The model under review builds one solid part; all positions refer to its coordinate system, in mm. A direction names the side the tool comes from. Give positions to 0.01 mm unless a question says otherwise; leave off trailing zeros. Loops run counter-clockwise (first coordinate to the right, second up) from the corner with the lowest first, then second, coordinate; pieces in that order, holes last. Notation, with made-up numbers: (8.25, -11) - (44.25, -11) arc R17 cw to (44.25, 9) - close; hole circle Ø4 at (-30.75, -3). An arc over 180 degrees is marked (long way). Return JSON: item names as keys, results as strings. Group by question number.
```python
from build123d import *

# Parameters (mm, degrees)
SKETCH1_W           = 172
SKETCH1_H           = 222
SKETCH1_R           = 1.55
SKETCH1_W_2         = 50
SKETCH1_H_2         = 10
BOSS_EXTRUDE2_DEPTH = 4
FILLET1_R           = 4


with BuildPart() as part:
    # Sketch1 → Boss-Extrude2 (new body)
    with BuildSketch(Plane(origin=(0, 0, 0), x_dir=(0, 1, 0), z_dir=(0, 0, 1))):
        with Locations((86, 111)):
            Rectangle(SKETCH1_W, SKETCH1_H)
        with Locations(Location((5, 4, 0), (0, 0, 270))):
            Circle(SKETCH1_R, mode=Mode.SUBTRACT)
        with Locations(Location((5, 218, 0), (0, 0, 270))):
            Circle(SKETCH1_R, mode=Mode.SUBTRACT)
        with Locations(Location((167, 218, 0), (0, 0, 270))):
            Circle(SKETCH1_R, mode=Mode.SUBTRACT)
        with Locations(Location((167, 4, 0), (0, 0, 270))):
            Circle(SKETCH1_R, mode=Mode.SUBTRACT)
        with Locations(Location((86, 218, 0), (0, 0, 270))):
            Circle(SKETCH1_R, mode=Mode.SUBTRACT)
        with Locations(Location((86, 4, 0), (0, 0, 270))):
            Circle(SKETCH1_R, mode=Mode.SUBTRACT)
        with Locations(Location((4, 61, 0), (0, 0, 270))):
            Circle(SKETCH1_R, mode=Mode.SUBTRACT)
        with Locations(Location((168, 61, 0), (0, 0, 270))):
            Circle(SKETCH1_R, mode=Mode.SUBTRACT)
        with Locations(Location((168, 161, 0), (0, 0, 270))):
            Circle(SKETCH1_R, mode=Mode.SUBTRACT)
        with Locations(Location((4, 161, 0), (0, 0, 270))):
            Circle(SKETCH1_R, mode=Mode.SUBTRACT)
        with Locations((55, 207)):
            Rectangle(SKETCH1_W_2, SKETCH1_H_2, mode=Mode.SUBTRACT)
        with Locations((55, 15)):
            Rectangle(SKETCH1_W_2, SKETCH1_H_2, mode=Mode.SUBTRACT)
        with BuildLine():
            Line((40, 131), (40, 91))
            ThreePointArc((40, 91), (35, 86), (30, 91))
            Line((30, 91), (30, 131))
            ThreePointArc((30, 131), (35, 136), (40, 131))
        make_face(mode=Mode.SUBTRACT)
        with BuildLine():
            Line((60, 131), (60, 91))
            ThreePointArc((60, 91), (55, 86), (50, 91))
            Line((50, 91), (50, 131))
            ThreePointArc((50, 131), (55, 136), (60, 131))
        make_face(mode=Mode.SUBTRACT)
        with BuildLine():
            Line((80, 131), (80, 91))
            ThreePointArc((80, 91), (75, 86), (70, 91))
            Line((70, 91), (70, 131))
            ThreePointArc((70, 131), (75, 136), (80, 131))
        make_face(mode=Mode.SUBTRACT)
        with BuildLine():
            Line((100, 131), (100, 91))
            ThreePointArc((100, 91), (95, 86), (90, 91))
            Line((90, 91), (90, 131))
            ThreePointArc((90, 131), (95, 136), (100, 131))
        make_face(mode=Mode.SUBTRACT)
        with BuildLine():
            Line((120, 131), (120, 91))
            ThreePointArc((120, 91), (115, 86), (110, 91))
            Line((110, 91), (110, 131))
            ThreePointArc((110, 131), (115, 136), (120, 131))
        make_face(mode=Mode.SUBTRACT)
        with BuildLine():
            Line((140, 131), (140, 91))
            ThreePointArc((140, 91), (135, 86), (130, 91))
            Line((130, 91), (130, 131))
            ThreePointArc((130, 131), (135, 136), (140, 131))
        make_face(mode=Mode.SUBTRACT)
    extrude(amount=BOSS_EXTRUDE2_DEPTH)

    # Fillet1
    # the kernel refuses this fillet: 4 mm, written as the material it takes off along each edge
    with BuildSketch(Plane(origin=(10, 172, 0), x_dir=(0, 0, 1), z_dir=(-1, 0, 0)), Plane(origin=(-232, 0, 0), x_dir=(0, 0, 1), z_dir=(1, 0, 0))) as fillet1_piece_1:
        with BuildLine():
            CenterArc((FILLET1_R, -FILLET1_R), FILLET1_R, 90, 90)
            Line((0, -FILLET1_R), (0, 0))
            Line((0, 0), (FILLET1_R, 0))
        make_face()
    extrude(amount=242, mode=Mode.SUBTRACT)


solid = part.part
```
1) We need section C-C, the plane y = 115. Write out the cut boundary in (x, z), plus the area to 3 significant figures.
2) We need section D-D, the plane z = 2.05. Count the separate pieces of the cut face and the enclosed holes in it, plus the area to 3 significant figures.
3) Draft analysis for pull direction X (two halves, no side actions). For faces 3 (the face through (-113, 85, 4)), 4 (the face through (-86, 95, 2)), 5 (the face through (-136, 55, 2)), state which applies: +X half, -X half, draft (parallel to the pull), parting line (faces both ways), or undercut.
4) We need section A-A, the plane x = -124. Write out the cut boundary in (y, z).
5) To check wall thickness, follow line 1 (X direction, y = 48.5, z = 3.35); line 2 (X direction, y = 167, z = 2.5); line 3 (Y direction, x = -218, z = 2.55). State the ranges of each line that lie inside material, in increasing order.
6) We need section B-B, the plane y = 55. Write out the cut boundary in (x, z).
7) For pin 1 Ø2 at (x, z) = (-118, 2) entering from +Y; pin 2 Ø2 at (x, z) = (-104, 1) entering from -Y; pin 3 Ø1.2 at (x, z) = (-118.5, 2.5) entering from -Y, all flat-tipped, find the tip position at first contact; note any pin that passes through.
8) Tool access review of faces 1 (the face through (-136, 115, 2)), 2 (the face through (-113, 85, 0)): name each direction out of +Z, -Z, +X, -X, +Y, -Y from which nothing blocks a thin tool from reaching the whole face with its end or side.
Findings:
{
 "1": {"outline": "(-222, 0) - (-136, 0) - (-136, 4) - (-222, 4) - close; (-86, 0) - (0, 0) - (0, 4) - (-86, 4) - close", "area": "688 mm^2"},
 "2": {"separate pieces": "1", "enclosed holes": "18", "area": "34,000 mm^2"},
 "3": {"face 3": "draft", "face 4": "undercut", "face 5": "undercut"},
 "4": {"outline": "(0, 4) arc R4 ccw to (4, 0) - (30, 0) - (30, 4) - close; (40, 0) - (50, 0) - (50, 4) - (40, 4) - close; (60, 0) - (70, 0) - (70, 4) - (60, 4) - close; (80, 0) - (90, 0) - (90, 4) - (80, 4) - close; (100, 0) - (110, 0) - (110, 4) - (100, 4) - close; (120, 0) - (130, 0) - (130, 4) - (120, 4) - close; (140, 0) - (168, 0) arc R4 ccw to (172, 4) - (140, 4) - close"},
 "5": {"line 1": "x = -222 to -212, -202 to -20, -10 to 0", "line 2": "x = -222 to -219.55, -216.45 to -162.18, -159.82 to -62.18, -59.82 to -5.55, -2.45 to 0", "line 3": "y = 0.27 to 3.45, 6.55 to 84.45, 87.55 to 165.45, 168.55 to 171.73"},
 "6": {"outline": "(-222, 0) - (-212, 0) - (-212, 4) - (-222, 4) - close; (-202, 0) - (-136, 0) - (-136, 4) - (-202, 4) - close; (-86, 0) - (-20, 0) - (-20, 4) - (-86, 4) - close; (-10, 0) - (0, 0) - (0, 4) - (-10, 4) - close"},
 "7": {"pin 1": "stops at y = 171.87", "pin 2": "stops at y = 0.54", "pin 3": "stops at y = 0.1"},
 "8": {"face 1": "+Z, -Z", "face 2": "-Z, +X, -X, +Y, -Y"}
}
